Could you check a few things on this model? Use its own coordinates, in mm. Face numbers are marked on the shaded views. A direction names the side the tool comes from. Round coordinates to 2 decimals unless told otherwise and drop trailing zeros. Put each result on its own line as item: value. Start each with the question number.
1. Which directions (+Z, -Z, +X, -X, +Y, -Y) give clear straight access to the entire face, cutting with the end or side of a thin tool? Please do the marked faces 1 and 2.
2. I need wall thicknesses on line 1 (X direction, y = 112, z = 4.25); line 2 (X direction, y = -0.5, z = 1.5); line 3 (X direction, y = 63, z = 1.25). Which ranges of each line are inside material? Lowest first, please. Write a range as [from, to].
3. Imagine slicing it at A-A, the plane z = 2.75. Count the separate pieces of the cut face and the enclosed holes in it, and give its area (3 significant figures).
4. I'm going to push flat-ended pins straight in: P1, Ø5, axis at y = 64, z = 11.5, coming from the +X side; P2, Ø5, axis at x = -15, z = 1.5, coming from the -Y side; P3, Ø4, axis at y = -14.5, z = 6, coming from the -X side. Where does each tip first touch, or does it pass through?
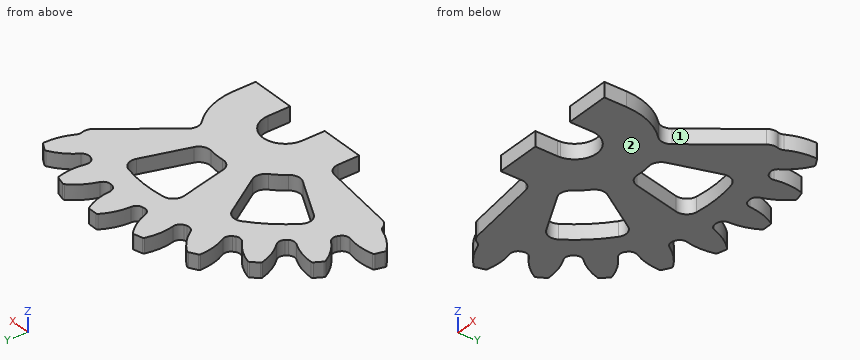
```python
from build123d import *

# Parameters (mm, degrees)
SKETCH3_R                = 136.611351841
EXTRUDE1_DEPTH           = 12.7
EXTRUDE2_DEPTH           = 12.7
FILLET2_R                = 1.5875
CIRPATTERN1_COUNT        = 24
FILLET2_OF_CIRPATTERN1_R = 1.5875
CUT_EXTRUDE1_DEPTH       = 234.890969431
CUT_EXTRUDE1_DEPTH_BACK  = 234.890969431
CUT_EXTRUDE2_REACH       = 232.646
SKETCH5_R                = 19.05
EXTRUDE3_DEPTH           = 12.7
CUT_EXTRUDE5_DEPTH       = 231.646456089
FILLET1_R                = 9.525
CUT_EXTRUDE7_DEPTH       = 12.7


with BuildPart() as part:
    # Sketch3 → Extrude1 (new body)
    with BuildSketch(Plane.XY):
        Circle(SKETCH3_R)
    extrude(amount=EXTRUDE1_DEPTH)

    # Sketch2 → Extrude2 (add)
    with BuildSketch(Plane.XY):
        with BuildLine():
            Line((-4.546074008, 165.141901983), (4.546074008, 165.141901983))
            ThreePointArc((4.546074008, 165.141901983), (9.719017906, 153.717756782), (11.846410355, 141.35876639))
            ThreePointArc((11.846410355, 141.35876639), (13.677789854, 137.226095775), (17.83135957, 135.442622788))
            Line((17.83135957, 135.442622788), (17.83135957, 110.042622788))
            Line((17.83135957, 110.042622788), (-17.83135957, 110.042622788))
            Line((-17.83135957, 110.042622788), (-17.83135957, 135.442622788))
            ThreePointArc((-17.83135957, 135.442622788), (-13.677789854, 137.226095775), (-11.846410355, 141.35876639))
            ThreePointArc((-11.846410355, 141.35876639), (-9.719017906, 153.717756782), (-4.546074008, 165.141901983))
        make_face()
    extrude2 = extrude(amount=EXTRUDE2_DEPTH)

    # Fillet2
    fillet2_edges = [part.edges().sort_by_distance(p)[0] for p in [
        (4.546074008, 165.141901983, 6.35),
        (-4.546074008, 165.141901983, 6.35),
    ]]
    fillet(fillet2_edges, radius=FILLET2_R)

    # CirPattern1: Extrude2 ×24 about axis
    cirpattern1_axis = Axis((0, 0, 0), (0, 0, 1))
    for i in range(1, CIRPATTERN1_COUNT):
        add(extrude2.rotate(cirpattern1_axis, i * 360 / CIRPATTERN1_COUNT))

    # Fillet2 of CirPattern1
    fillet2_of_cirpattern1_edges = [part.edges().sort_by_distance(p)[0] for p in [
        (-38.350699085, 160.691438662, 6.35),
        (-47.13303967, 158.338217595, 6.35),
        (-78.633935413, 145.290119351, 6.35),
        (-86.50796657, 140.744045343, 6.35),
        (-113.558398992, 119.987518509, 6.35),
        (-119.987518509, 113.558398992, 6.35),
        (-140.744045343, 86.50796657, 6.35),
        (-145.290119351, 78.633935413, 6.35),
        (-158.338217595, 47.13303967, 6.35),
        (-160.691438662, 38.350699085, 6.35),
        (-165.141901983, 4.546074008, 6.35),
        (-165.141901983, -4.546074008, 6.35),
        (-160.691438662, -38.350699085, 6.35),
        (-158.338217595, -47.13303967, 6.35),
        (-145.290119351, -78.633935413, 6.35),
        (-140.744045343, -86.50796657, 6.35),
        (-119.987518509, -113.558398992, 6.35),
        (-113.558398992, -119.987518509, 6.35),
        (-86.50796657, -140.744045343, 6.35),
        (-78.633935413, -145.290119351, 6.35),
        (-47.13303967, -158.338217595, 6.35),
        (-38.350699085, -160.691438662, 6.35),
        (-4.546074008, -165.141901983, 6.35),
        (4.546074008, -165.141901983, 6.35),
        (38.350699085, -160.691438662, 6.35),
        (47.13303967, -158.338217595, 6.35),
        (78.633935413, -145.290119351, 6.35),
        (86.50796657, -140.744045343, 6.35),
        (113.558398992, -119.987518509, 6.35),
        (119.987518509, -113.558398992, 6.35),
        (140.744045343, -86.50796657, 6.35),
        (145.290119351, -78.633935413, 6.35),
        (158.338217595, -47.13303967, 6.35),
        (160.691438662, -38.350699085, 6.35),
        (165.141901983, -4.546074008, 6.35),
        (165.141901983, 4.546074008, 6.35),
        (160.691438662, 38.350699085, 6.35),
        (158.338217595, 47.13303967, 6.35),
        (145.290119351, 78.633935413, 6.35),
        (140.744045343, 86.50796657, 6.35),
        (119.987518509, 113.558398992, 6.35),
        (113.558398992, 119.987518509, 6.35),
        (86.50796657, 140.744045343, 6.35),
        (78.633935413, 145.290119351, 6.35),
        (47.13303967, 158.338217595, 6.35),
        (38.350699085, 160.691438662, 6.35),
    ]]
    fillet(fillet2_of_cirpattern1_edges, radius=FILLET2_OF_CIRPATTERN1_R)

    # Sketch4 → Cut-Extrude1 (cut, two sides: drawn at the far end of the back side and taken through both)
    with BuildSketch(Plane.XY.offset(-CUT_EXTRUDE1_DEPTH_BACK)):
        Polygon((-1275.53694573, 167.92762467), (-268.218413087, 35.311623982), (0, 0), (164.689969961, 214.628147505), (783.198061827, 1020.683586133), (1560.818943381, -856.6592925), (-497.916064176, -1709.415253962), align=None)
    extrude(amount=CUT_EXTRUDE1_DEPTH + CUT_EXTRUDE1_DEPTH_BACK, mode=Mode.SUBTRACT)

    # Sketch5 → Cut-Extrude2 (cut, up to next)
    with BuildSketch(Plane.XY, mode=Mode.PRIVATE) as cut_extrude2_sk1:
        Circle(SKETCH5_R)
    cut_extrude2_tool1 = extrude(cut_extrude2_sk1.sketch, amount=CUT_EXTRUDE2_REACH, mode=Mode.PRIVATE) & part.part
    add(cut_extrude2_tool1.solids().sort_by_distance((0, 0, 0))[0], mode=Mode.SUBTRACT)

    # Sketch6 → Extrude3 (add)
    with BuildSketch(Plane.XY):
        with BuildLine():
            Line((-19.05, 0), (-19.05, -19.05))
            Line((-19.05, -19.05), (-57.15, -19.05))
            Line((-57.15, -19.05), (-57.15, 0))
            ThreePointArc((-57.15, 0), (-57.027637463, 3.737788836), (-56.661073828, 7.459571885))
            Line((-56.661073828, 7.459571885), (-18.887024609, 2.486523962))
            ThreePointArc((-18.887024609, 2.486523962), (-19.009212488, 1.245929612), (-19.05, 0))
        make_face()
        with BuildLine():
            Line((11.596905223, 15.113381133), (34.790715668, 45.340143398))
            ThreePointArc((34.790715668, 45.340143398), (51.256277179, 25.276798646), (57.15, 0))
            Line((57.15, 0), (57.15, -19.05))
            Line((57.15, -19.05), (19.05, -19.05))
            Line((19.05, -19.05), (19.05, 0))
            ThreePointArc((19.05, 0), (17.085425726, 8.425599549), (11.596905223, 15.113381133))
        make_face()
    extrude(amount=EXTRUDE3_DEPTH)

    # Sketch8 → Cut-Extrude5 (cut, through all)
    with BuildSketch(Plane.XY):
        with BuildLine():
            Line((-25.426243647, 114.690373436), (-12.369523937, 55.795316807))
            ThreePointArc((-12.369523937, 55.795316807), (2.492847988, 57.095605863), (17.185336442, 54.504923735))
            Line((17.185336442, 54.504923735), (35.325413797, 112.037898789))
            ThreePointArc((35.325413797, 112.037898789), (5.124187531, 117.36318983), (-25.426243647, 114.690373436))
        make_face()
        with BuildLine():
            Line((-63.119271491, 99.077410097), (-30.706672617, 48.199821128))
            ThreePointArc((-30.706672617, 48.199821128), (-42.135399799, 38.609980365), (-50.692669116, 26.388933246))
            Line((-50.692669116, 26.388933246), (-104.201597628, 54.24391834))
            ThreePointArc((-104.201597628, 54.24391834), (-86.611655142, 79.36495964), (-63.119271491, 99.077410097))
        make_face()
    extrude(amount=CUT_EXTRUDE5_DEPTH, mode=Mode.SUBTRACT)

    # Fillet1
    fillet1_edges = [part.edges().sort_by_distance(p)[0] for p in [
        (34.790715668, 45.340143398, 6.35),
        (-50.692669116, 26.388933246, 6.35),
        (-30.706672617, 48.199821128, 6.35),
        (-63.119271491, 99.077410097, 6.35),
        (-104.201597628, 54.24391834, 6.35),
        (-12.369523937, 55.795316807, 6.35),
        (17.185336442, 54.504923735, 6.35),
        (35.325413797, 112.037898789, 6.35),
        (-25.426243647, 114.690373436, 6.35),
        (-56.661073828, 7.459571885, 6.35),
        (-57.15, 0, 6.35),
    ]]
    fillet(fillet1_edges, radius=FILLET1_R)

    # Sketch9 → Cut-Extrude7 (cut)
    with BuildSketch(Plane.XY):
        with BuildLine():
            Line((79.034097122, 102.999240689), (83.809524096, 109.222698287))
            Line((83.809524096, 109.222698287), (80.539107883, 111.732176909))
            ThreePointArc((80.539107883, 111.732176909), (80.864034333, 107.180027092), (79.034097122, 102.999240689))
        make_face()
        with BuildLine():
            Line((-128.717007568, 16.945915528), (-136.494393434, 17.969827802))
            Line((-136.494393434, 17.969827802), (-135.956329304, 22.056830634))
            ThreePointArc((-135.956329304, 22.056830634), (-132.967230996, 18.608216933), (-128.717007568, 16.945915528))
        make_face()
    extrude(amount=CUT_EXTRUDE7_DEPTH, mode=Mode.SUBTRACT)


solid = part.part
```
Entries:
1. face 1: +Z, -Z, +X
1. face 2: -Z, +X, -X, +Y, -Y
2. line 1: [-119.59, -96.08], [-80.46, -22.11], [30.13, 80.46]
2. line 2: [-57.16, -19.05], [19.05, 57.15]
2. line 3: [-132.02, -99.15], [-40.14, -13.85], [19.86, 48.34]
3. separate pieces: 1
3. enclosed holes: 2
3. area: 21,400 mm^2
4. P1: x = 51.03
4. P2: y = 7.53
4. P3: x = -57.15
